Read the model definition and answer for the solid it produces. Units are mm, in the model's axes. A direction names the side the tool comes from. Round coordinates to 2 decimals unless told otherwise and drop trailing zeros. Loops run counter-clockwise (first coordinate to the right, second up) from the corner with the lowest first, then second, coordinate; pieces in that order, holes last. Notation, with made-up numbers: (8.25, -37) - (57.25, -37) arc R27 ccw to (57.25, 1) - close; hole circle Ø6 at (70.5, -13). An arc over 180 degrees is marked (long way). Use CSV: the item, a comma, the result in double quotes. Start each with the question number.
1. Find section D-D (x = 29). Give the vertices of the cut face in (y, z), and give its area (3 significant figures).
2. Given pin 1 Ø2 at (x, y) = (31, -5) entering from -Z; pin 2 Ø6 at (y, z) = (7.5, -1.5) entering from +X; pin 3 Ø5 at (y, z) = (9, -15) entering from -X, each flat-ended and moving along its own axis, determine where each tip first touches the part or whether it passes through.
3. Consider line 1 along X through (y, z) = (-4.75, -8.5); line 2 along X through (y, z) = (6.5, -7); line 3 along Z through (x, y) = (32.75, 9.5). Determine where each line is inside the solid, lowest interval first.
4. Find section B-B (x = 38.25). Give the vertices of the cut face in (y, z).
5. Determine the mould class of faces 3 (the cylindrical face through (32.537, -0.173, -9.86)), 4 (the cylindrical face through (35.834, 0.178, -8.661)), 5 (the flat face through (28, 0, -20)) for opening direction Y: +Y half, -Y half, draft (parallel to the pull), parting line (faces both ways), or undercut.
6. Find section C-C (y = 6). Give the vertices of the cut face in (x, z), and give its area (3 significant figures).
7. A tool of negligible diameter and unlimited length cuts with its end or side. For faces 1 (the cylindrical face through (28.344, -0.179, -9.86)), 2 (the flat face through (35, 0, -20)), from which of +Z, -Z, +X, -X, +Y, -Y can it reach the whole face along a straight path? Write none if from no direction.
8. Find section A-A (z = -8.75). Give the vertices of the cut face in (x, y).
from build123d import *

# Parameters (mm, degrees)
BOSS_EXTRUDE1_DEPTH = 3
BOSS_EXTRUDE2_DEPTH = 20


with BuildPart() as part:
    # Sketch1 → Boss-Extrude1 (new body)
    with BuildSketch(Plane.XY):
        with BuildLine():
            ThreePointArc((28.476711912, -13.065389126), (26.043422294, 0), (28.476711912, 13.065389126))
            ThreePointArc((28.476711912, 13.065389126), (33.603633576, 12.069057908), (38.823996353, 12.229725621))
            ThreePointArc((38.823996353, 12.229725621), (35.833644105, 0), (38.823996353, -12.229725621))
            ThreePointArc((38.823996353, -12.229725621), (33.603633576, -12.069057908), (28.476711912, -13.065389126))
        make_face()
    extrude(amount=BOSS_EXTRUDE1_DEPTH)

    # Sketch2 → Boss-Extrude2 (add)
    with BuildSketch(Plane(origin=(0, 0, 0), x_dir=(-1, 0, 0), z_dir=(0, 0, -1))):
        with BuildLine():
            ThreePointArc((-30.718530844, -12.483407407), (-28.343422286, 0), (-30.718530844, 12.483407407))
            ThreePointArc((-30.718530844, 12.483407407), (-29.5904471, 12.746762635), (-28.476711912, 13.065389126))
            ThreePointArc((-28.476711912, 13.065389126), (-26.043422294, 0), (-28.476711912, -13.065389126))
            ThreePointArc((-28.476711912, -13.065389126), (-29.5904471, -12.746762635), (-30.718530844, -12.483407407))
        make_face()
        with BuildLine():
            ThreePointArc((-38.823996353, 12.229725621), (-35.833644105, 0), (-38.823996353, -12.229725621))
            ThreePointArc((-38.823996353, -12.229725621), (-36.94579852, -12.037595161), (-35.058238797, -11.996858122))
            ThreePointArc((-35.058238797, -11.996858122), (-32.536736444, 0), (-35.058238797, 11.996858122))
            ThreePointArc((-35.058238797, 11.996858122), (-36.94579852, 12.037595161), (-38.823996353, 12.229725621))
        make_face()
    extrude(amount=BOSS_EXTRUDE2_DEPTH)


solid = part.part
Filled sheet:
1,outline,"(-12.91, -20) - (-6.65, -20) - (-6.65, 0) - (6.65, 0) - (6.65, -20) - (12.91, -20) - (12.91, 3) - (-12.91, 3) - close"
1,area,"328 mm²"
2,pin 1,"stops at z = 0"
2,pin 2,"stops at x = 38"
2,pin 3,"stops at x = 26.63"
3,line 1,"x = 26.36 to 28.68, 32.92 to 36.26"
3,line 2,"x = 26.63 to 28.97, 33.25 to 36.64"
3,line 3,"z = 0 to 3"
4,outline,"(-12.15, -20) - (-11.06, -20) - (-11.06, 3) - (-12.15, 3) - close; (11.06, -20) - (12.15, -20) - (12.15, 3) - (11.06, 3) - close"
5,face 3,"parting line"
5,face 4,"undercut"
5,face 5,"draft"
6,outline,"(26.54, -20) - (28.88, -20) - (28.88, 0) - (33.15, 0) - (33.15, -20) - (36.52, -20) - (36.52, 3) - (26.54, 3) - close"
6,area,"144 mm²"
7,face 1,"-Z"
7,face 2,"-Z, +X, -X, +Y, -Y"
8,outline,"(28.48, -13.07) arc R23.5 cw to (30.72, -12.48) arc R33.99 cw to (30.72, 12.48) arc R23.5 cw to (28.48, 13.07) arc R36.29 ccw to start; (35.06, -12) arc R23.5 cw to (38.82, -12.23) arc R26.5 cw to (38.82, 12.23) arc R23.5 cw to (35.06, 12) arc R29.8 ccw to start"
